```python
from build123d import *

# Parameters (mm, degrees)
BOSS_EXTRUDE1_DEPTH = 20
SKETCH2_R           = 4
SKETCH2_R_2         = 2
BOSS_EXTRUDE2_DEPTH = 5
SKETCH2_4_R         = 2
BOSS_EXTRUDE3_DEPTH = 10
SKETCH3_R           = 4
SKETCH3_R_2         = 1.75
BOSS_EXTRUDE4_DEPTH = 5
SKETCH3_2_R         = 1.75
BOSS_EXTRUDE5_DEPTH = 10
BOSS_EXTRUDE6_START = 5
SKETCH4_R           = 4
SKETCH4_R_2         = 2.25
BOSS_EXTRUDE6_DEPTH = 5
BOSS_EXTRUDE7_START = 10
SKETCH4_2_R         = 2.25
BOSS_EXTRUDE7_DEPTH = 10
CHAMFER1_SIZE       = 3.03
CHAMFER1_SIZE2      = 1.749371316
CHAMFER2_SIZE       = 3.46
CHAMFER2_SIZE2      = 1.997631931
CHAMFER3_SIZE       = 3.89
CHAMFER3_SIZE2      = 2.245892547
CHAMFER4_SIZE       = 1


with BuildPart() as part:
    # Sketch1 → Boss-Extrude1 (new body)
    with BuildSketch(Plane(origin=(0, 0, 0), x_dir=(1, 0, 0), z_dir=(0, 1, 0))):
        Polygon((-42.5, 0), (-42.5, -20), (42.5, -20), (42.5, 0), (7.5, 0), (7.5, 20), (-7.5, 20), (-7.5, 0), align=None)
    extrude(amount=BOSS_EXTRUDE1_DEPTH)

    # Sketch2 → Boss-Extrude2 (add)
    with BuildSketch(Plane(origin=(0, 0, -20), x_dir=(-1, 0, 0), z_dir=(0, 0, -1))):
        with Locations(Location((0, 10, 0), (0, 0, 180))):
            Circle(SKETCH2_R)
        with Locations((0, 10)):
            Circle(SKETCH2_R_2, mode=Mode.SUBTRACT)
    extrude(amount=BOSS_EXTRUDE2_DEPTH)

    # Sketch2_4 → Boss-Extrude3 (add)
    with BuildSketch(Plane(origin=(0, 0, -20), x_dir=(-1, 0, 0), z_dir=(0, 0, -1))):
        with Locations((0, 10)):
            Circle(SKETCH2_4_R)
    extrude(amount=BOSS_EXTRUDE3_DEPTH)

    # Sketch3 → Boss-Extrude4 (add)
    with BuildSketch(Plane.ZY.offset(42.5)):
        with Locations((10, 10)):
            Circle(SKETCH3_R)
        with Locations((10, 10)):
            Circle(SKETCH3_R_2, mode=Mode.SUBTRACT)
    extrude(amount=BOSS_EXTRUDE4_DEPTH)

    # Sketch3_2 → Boss-Extrude5 (add)
    with BuildSketch(Plane.ZY.offset(42.5)):
        with Locations((10, 10)):
            Circle(SKETCH3_2_R)
    extrude(amount=BOSS_EXTRUDE5_DEPTH)

    # Sketch4 → Boss-Extrude6 (add)
    with BuildSketch(Plane(origin=(42.5, 0, 0), x_dir=(0, 0, -1), z_dir=(1, 0, 0)).offset(BOSS_EXTRUDE6_START)):
        with Locations(Location((-10, 10, 0), (0, 0, 180))):
            Circle(SKETCH4_R)
        with Locations((-10, 10)):
            Circle(SKETCH4_R_2, mode=Mode.SUBTRACT)
    extrude(amount=-BOSS_EXTRUDE6_DEPTH)

    # Sketch4_2 → Boss-Extrude7 (add)
    with BuildSketch(Plane(origin=(42.5, 0, 0), x_dir=(0, 0, -1), z_dir=(1, 0, 0)).offset(BOSS_EXTRUDE7_START)):
        with Locations((-10, 10)):
            Circle(SKETCH4_2_R)
    extrude(amount=-BOSS_EXTRUDE7_DEPTH)

    # Chamfer1
    chamfer1_edges = [part.edges().sort_by_distance(p)[0] for p in [
        (-52.5, 10, 8.25),
    ]]
    chamfer1_side = [part.faces().sort_by_distance(p)[0] for p in [
        (-50, 10, 8.25),
    ]]
    chamfer(chamfer1_edges, length=CHAMFER1_SIZE, length2=CHAMFER1_SIZE2, reference=chamfer1_side[0])

    # Chamfer2
    chamfer2_edges = [part.edges().sort_by_distance(p)[0] for p in [
        (2, 10, -30),
    ]]
    chamfer2_side = [part.faces().sort_by_distance(p)[0] for p in [
        (2, 10, -27.5),
    ]]
    chamfer(chamfer2_edges, length=CHAMFER2_SIZE, length2=CHAMFER2_SIZE2, reference=chamfer2_side[0])

    # Chamfer3
    chamfer3_edges = [part.edges().sort_by_distance(p)[0] for p in [
        (52.5, 10, 12.25),
    ]]
    chamfer3_side = [part.faces().sort_by_distance(p)[0] for p in [
        (50, 10, 12.25),
    ]]
    chamfer(chamfer3_edges, length=CHAMFER3_SIZE, length2=CHAMFER3_SIZE2, reference=chamfer3_side[0])

    # Chamfer4
    chamfer4_edges = [part.edges().sort_by_distance(p)[0] for p in [
        (7.5, 0, -10),
        (25, 0, 0),
        (42.5, 0, 10),
        (0, 0, 20),
        (25, 20, 0),
        (-42.5, 10, 20),
        (-42.5, 10, 0),
        (-7.5, 10, 0),
        (-7.5, 10, -20),
        (7.5, 10, -20),
        (7.5, 10, 0),
        (42.5, 10, 0),
        (42.5, 10, 20),
        (7.5, 20, -10),
        (0, 20, -20),
        (-4, 10, -20),
        (-7.5, 20, -10),
        (-4, 10, -25),
        (-25, 20, 0),
        (-42.5, 20, 10),
        (-42.5, 10, 6),
        (-47.5, 10, 6),
        (42.5, 10, 6),
        (47.5, 10, 6),
        (0, 20, 20),
        (-42.5, 0, 10),
        (42.5, 20, 10),
        (-25, 0, 0),
        (-7.5, 0, -10),
        (0, 0, -20),
    ]]
    chamfer(chamfer4_edges, length=CHAMFER4_SIZE)


solid = part.part
```
Could you check a few things on this model? Use its own coordinates, in mm. A direction names the side the tool comes from. Coordinates: 2 decimals unless noted, no trailing zeros. Loops run counter-clockwise (first coordinate to the right, second up) from the corner with the lowest first, then second, coordinate; pieces in that order, holes last. Notation, with made-up numbers: M -14.5,-10 L 14.5,-10 A25 ccw 14.5,8 Z; hole C 85,4 d10. An arc over 180 degrees is marked long. Put each result on its own line as item: value. Start each with the question number.
(1) Suppose I cut it at C-C on z = -6. Please give me the cut outline in (x, y).
(2) Suppose I cut it at A-A on y = 4. Please give me the cut outline in (x, z), then the cut area to 3 significant figures.
(3) Suppose I cut it at B-B on x = -39.5. Please give me the cut outline in (y, z).
(4) Suppose I cut it at D-D on z = -22. Please give me the cut outline in (x, y).
(5) I need wall thicknesses on line 1 (X direction, y = 6.75, z = -13.5); line 2 (X direction, y = 9.5, z = 17); line 3 (Z direction, x = 5.5, y = 2). Which ranges of each line are inside material? Lowest first, please. Write a range as from..to.
(6) Will these pins go through, and if not, where does the flat tip stop? P1, Ø5.5, axis at y = 10.5, z = -9, coming from the +X side; P2, Ø2, axis at y = 15, z = 8.5, coming from the +X side; P3, Ø2, axis at x = -12.5, y = 9, coming from the -Z side.
(7) For faces 1 (the face through (-7.5, 10, -10)), 2 (the face through (0, 12, -26)), 3 (the face through (48.06, 11.52, 11.66)), which set-ups out of +Z, -Z, +X, -X, +Y, -Y let a thin tool reach every point of the face, with its end or its side?
Solutions:
1. outline: M -7.5,1 L -6.5,0 L 6.5,0 L 7.5,1 L 7.5,19 L 6.5,20 L -6.5,20 L -7.5,19 Z
2. outline: M -42.5,1 L -41.5,0 L -8.5,0 L -7.5,-1 L -7.5,-19 L -6.5,-20 L 6.5,-20 L 7.5,-19 L 7.5,-1 L 8.5,0 L 41.5,0 L 42.5,1 L 42.5,19 L 41.5,20 L -41.5,20 L -42.5,19 Z
2. area: 2,000 mm2
3. outline: M 0,1 L 1,0 L 19,0 L 20,1 L 20,19 L 19,20 L 1,20 L 0,19 Z
4. outline: C 0,10 d8
5. line 1: x = -7.5..7.5
5. line 2: x = -42.5..42.5
5. line 3: z = -20..20
6. P1: stops at x = 7.5
6. P2: stops at x = 43.28
6. P3: stops at z = 0
7. face 1: -Z, -X, +Y, -Y
7. face 2: -Z
7. face 3: +X
